```python
from build123d import *

# Parameters (mm, degrees)
SKETCH1_W           = 80
SKETCH1_H           = 67
SKETCH1_R           = 2.25
BOSS_EXTRUDE1_DEPTH = 2


with BuildPart() as part:
    # Sketch1 → Boss-Extrude1 (new body)
    with BuildSketch(Plane(origin=(0, 0, 0), x_dir=(1, 0, 0), z_dir=(0, 1, 0))):
        with Locations((-5, 2.5)):
            Rectangle(SKETCH1_W, SKETCH1_H)
        with Locations((30, -26)):
            Circle(SKETCH1_R, mode=Mode.SUBTRACT)
        with Locations((-40, -26)):
            Circle(SKETCH1_R, mode=Mode.SUBTRACT)
        with Locations((-40, 31)):
            Circle(SKETCH1_R, mode=Mode.SUBTRACT)
        with Locations((30, 31)):
            Circle(SKETCH1_R, mode=Mode.SUBTRACT)
        with BuildLine():
            Line((-22.02081528, 13.62081528), (-12.02081528, 13.62081528))
            ThreePointArc((-12.02081528, 13.62081528), (-10.42081528, 12.02081528), (-12.02081528, 10.42081528))
            Line((-12.02081528, 10.42081528), (-22.02081528, 10.42081528))
            ThreePointArc((-22.02081528, 10.42081528), (-23.62081528, 12.02081528), (-22.02081528, 13.62081528))
        make_face(mode=Mode.SUBTRACT)
        with BuildLine():
            Line((2.02081528, 13.62081528), (12.02081528, 13.62081528))
            ThreePointArc((12.02081528, 13.62081528), (13.62081528, 12.02081528), (12.02081528, 10.42081528))
            Line((12.02081528, 10.42081528), (2.02081528, 10.42081528))
            ThreePointArc((2.02081528, 10.42081528), (0.42081528, 12.02081528), (2.02081528, 13.62081528))
        make_face(mode=Mode.SUBTRACT)
        with BuildLine():
            Line((-10, 5), (0, 5))
            ThreePointArc((0, 5), (5, 0), (0, -5))
            Line((0, -5), (-10, -5))
            ThreePointArc((-10, -5), (-15, 0), (-10, 5))
        make_face(mode=Mode.SUBTRACT)
        with BuildLine():
            Line((-22.02081528, -13.62081528), (-12.02081528, -13.62081528))
            ThreePointArc((-12.02081528, -13.62081528), (-10.42081528, -12.02081528), (-12.02081528, -10.42081528))
            Line((-12.02081528, -10.42081528), (-22.02081528, -10.42081528))
            ThreePointArc((-22.02081528, -10.42081528), (-23.62081528, -12.02081528), (-22.02081528, -13.62081528))
        make_face(mode=Mode.SUBTRACT)
        with BuildLine():
            Line((2.02081528, -13.62081528), (12.02081528, -13.62081528))
            ThreePointArc((12.02081528, -13.62081528), (13.62081528, -12.02081528), (12.02081528, -10.42081528))
            Line((12.02081528, -10.42081528), (2.02081528, -10.42081528))
            ThreePointArc((2.02081528, -10.42081528), (0.42081528, -12.02081528), (2.02081528, -13.62081528))
        make_face(mode=Mode.SUBTRACT)
    extrude(amount=BOSS_EXTRUDE1_DEPTH)


solid = part.part
```
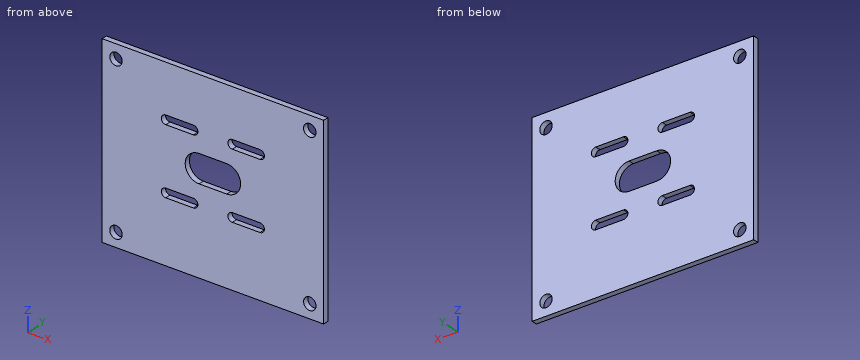
Geometry: final body of the model. Coordinates: model frame, mm. Coordinates: 2 decimals unless noted, no trailing zeros. Loops run counter-clockwise (first coordinate to the right, second up) from the corner with the lowest first, then second, coordinate; pieces in that order, holes last. Notation, with made-up numbers: M 48.25,0.25 L 61.25,0.25 A32 ccw 61.25,32.25 Z; hole C 69,79 d4. An arc over 180 degrees is marked long. Put each result on its own line as item: value.
(1) Cut plane A-A on z = 26. Return the cut outline in (x, y).
Answer sheet:
outline: M -45,0 L -42.25,0 L -42.25,2 L -45,2 Z; M -37.75,0 L 27.75,0 L 27.75,2 L -37.75,2 Z; M 32.25,0 L 35,0 L 35,2 L 32.25,2 Z
(2) Cut plane C-C on x = -19. Return the cut outline in (y, z).
Answer sheet:
outline: M 0,-36 L 2,-36 L 2,-13.62 L 0,-13.62 Z; M 0,-10.42 L 2,-10.42 L 2,10.42 L 0,10.42 Z; M 0,13.62 L 2,13.62 L 2,31 L 0,31 Z
(3) Cut plane B-B on y = 1.6. State how many separate pieces and enclosed holes the cut face has, then the cut area to 3 significant figures.
Answer sheet:
separate pieces: 1
enclosed holes: 9
area: 4,960 mm^2
(4) Material intervals for probe 1 along X at (y, z) = (0.1, -12); probe 2 along Z at (x, y) = (30, 1.2); probe 3 along X at (y, z) = (1.15, -31), sorted ascending.
Answer sheet:
probe 1: x = -45 to -23.62, -10.42 to 0.42, 13.62 to 35
probe 2: z = -36 to -33.25, -28.75 to 23.75, 28.25 to 31
probe 3: x = -45 to -42.25, -37.75 to 27.75, 32.25 to 35
(5) First-contact query: pin 1 (4 mm diameter, centred on x = -40, z = -31, fed in from -Y). Flat tip, straight axial feed; report the tip coordinate or a pass-through.
Answer sheet:
pin 1: passes through
(6) Cut plane D-D on z = 4. Return the cut outline in (x, y), then the cut area to 3 significant figures.
Answer sheet:
outline: M -45,0 L -13,0 L -13,2 L -45,2 Z; M 3,0 L 35,0 L 35,2 L 3,2 Z
area: 128 mm^2
